```python
from build123d import *
from build123d.topology import SkipClean

# Parameters (mm, degrees)
SKETCH1_R      = 10.5
EXTRUDE1_DEPTH = 1
EXTRUDE6_DEPTH = 3
SKETCH9_R      = 5.75
EXTRUDE9_DEPTH = 0.25
SKETCH7_R      = 4.9
EXTRUDE7_DEPTH = 2.366666667
SKETCH8_R      = 2
EXTRUDE8_DEPTH = 17.156560415
FILLET2_R      = 0.4
CHAMFER2_SIZE  = 1
FILLET3_R      = 1.5


with BuildPart() as part:
    # Sketch1 → Extrude1 (new body)
    with BuildSketch(Plane(origin=(0, 0, 0), x_dir=(1, 0, 0), z_dir=(0, 1, 0))):
        with Locations(Location((0, 0, 0), (0, 0, 270))):
            Circle(SKETCH1_R)
    extrude(amount=EXTRUDE1_DEPTH)

    # Sketch6 → Extrude6 (add)
    with SkipClean():  # the faces are left unmerged after this step: merging them gives an invalid solid
        with BuildSketch(Plane(origin=(0, 1, 0), x_dir=(1, 0, 0), z_dir=(0, 1, 0))):
            with BuildLine():
                Line((-2, 10.307764064), (-2, 8.209902557))
                ThreePointArc((-2, 8.209902557), (-5.975052301, 5.975052301), (-8.209902557, 2))
                Line((-8.209902557, 2), (-10.307764064, 2))
                ThreePointArc((-10.307764064, 2), (-7.424621202, 7.424621202), (-2, 10.307764064))
            make_face()
            with BuildLine():
                Line((2, 10.307764064), (2, 8.209902557))
                ThreePointArc((2, 8.209902557), (5.975052301, 5.975052301), (8.209902557, 2))
                Line((8.209902557, 2), (10.307764064, 2))
                ThreePointArc((10.307764064, 2), (7.424621202, 7.424621202), (2, 10.307764064))
            make_face()
            with BuildLine():
                Line((10.307764064, -2), (8.209902557, -2))
                ThreePointArc((8.209902557, -2), (5.975052301, -5.975052301), (2, -8.209902557))
                Line((2, -8.209902557), (2, -10.307764064))
                ThreePointArc((2, -10.307764064), (7.424621202, -7.424621202), (10.307764064, -2))
            make_face()
            with BuildLine():
                Line((-2, -10.307764064), (-2, -8.209902557))
                ThreePointArc((-2, -8.209902557), (-5.975052301, -5.975052301), (-8.209902557, -2))
                Line((-8.209902557, -2), (-10.307764064, -2))
                ThreePointArc((-10.307764064, -2), (-7.424621202, -7.424621202), (-2, -10.307764064))
            make_face()
        extrude(amount=EXTRUDE6_DEPTH)

    # Sketch9 → Extrude9 (cut)
    with SkipClean():  # the faces are left unmerged after this step: merging them gives an invalid solid
        with BuildSketch(Plane(origin=(0, 1, 0), x_dir=(1, 0, 0), z_dir=(0, 1, 0))):
            with Locations(Location((0, 0, 0), (0, 0, 270))):
                Circle(SKETCH9_R)
        extrude(amount=-EXTRUDE9_DEPTH, mode=Mode.SUBTRACT)

    # Sketch7 → Extrude7 (add)
    with SkipClean():  # the faces are left unmerged after this step: merging them gives an invalid solid
        with BuildSketch(Plane.XZ):
            with Locations(Location((0, 0, 0), (0, 0, 270))):
                Circle(SKETCH7_R)
        extrude(amount=EXTRUDE7_DEPTH)

    # Sketch8 → Extrude8 (cut, through all)
    with SkipClean():  # the faces are left unmerged after this step: merging them gives an invalid solid
        with BuildSketch(Plane.XZ.offset(2.366666667)):
            with Locations(Location((0, 0, 0), (0, 0, 270))):
                Circle(SKETCH8_R)
        extrude(amount=-EXTRUDE8_DEPTH, mode=Mode.SUBTRACT)

    # Fillet2
    fillet2_edges = [part.edges().sort_by_distance(p)[0] for p in [
        (5.975052301, 4, -5.975052301),
        (5.975052301, 4, 5.975052301),
        (-5.975052301, 4, 5.975052301),
        (0, -2.366666667, 4.9),
        (-5.975052301, 4, -5.975052301),
    ]]
    fillet(fillet2_edges, radius=FILLET2_R)

    # Chamfer2
    chamfer2_edges = [part.edges().sort_by_distance(p)[0] for p in [
        (0, -2.366666667, 2),
    ]]
    chamfer(chamfer2_edges, length=CHAMFER2_SIZE)

    # Fillet3
    # the kernel refuses this fillet: 1.5 mm, written as the material it adds along each edge
    with BuildSketch(Plane(origin=(2, 1, -14.057764064), x_dir=(-1, 0, 0), z_dir=(0, 0, 1))) as fillet3_piece_1_section:
        with BuildLine():
            CenterArc((FILLET3_R, -FILLET3_R), FILLET3_R, 90, 90)
            Line((0, -FILLET3_R), (0, 0))
            Line((0, 0), (FILLET3_R, 0))
        make_face()
    fillet3_piece_1 = extrude(amount=9.597861507, mode=Mode.PRIVATE)
    fillet3_piece_1 = fillet3_piece_1 & Plane(origin=(0, 1.340711746, 0), x_dir=(0, 0, 1), z_dir=(0, -1, 0)) * Cylinder(10.5, 26, mode=Mode.PRIVATE)
    fillet3_piece_1 = fillet3_piece_1 - Plane(origin=(0, 1.340711746, 0), x_dir=(0.23668639053254556, 0, -0.9715861014530186), z_dir=(0, -1, 0)) * Cylinder(8.45, 26, mode=Mode.PRIVATE)
    with BuildSketch(Plane(origin=(4.459902557, 1, -2), x_dir=(0, 0, 1), z_dir=(1, 0, 0))) as fillet3_piece_2_section:
        with BuildLine():
            CenterArc((FILLET3_R, -FILLET3_R), FILLET3_R, 90, 90)
            Line((0, -FILLET3_R), (0, 0))
            Line((0, 0), (FILLET3_R, 0))
        make_face()
    fillet3_piece_2 = extrude(amount=9.597861507, mode=Mode.PRIVATE)
    fillet3_piece_2 = fillet3_piece_2 & Plane(origin=(0, 1.34071094, 0), x_dir=(0, 0, 1), z_dir=(0, -1, 0)) * Cylinder(10.5, 26, mode=Mode.PRIVATE)
    fillet3_piece_2 = fillet3_piece_2 - Plane(origin=(0, 1.34071094, 0), x_dir=(0.23668639053254556, 0, -0.9715861014530186), z_dir=(0, -1, 0)) * Cylinder(8.45, 26, mode=Mode.PRIVATE)
    with BuildSketch(Plane(origin=(14.057764064, 1, 2), x_dir=(0, 0, -1), z_dir=(-1, 0, 0))) as fillet3_piece_3_section:
        with BuildLine():
            CenterArc((FILLET3_R, -FILLET3_R), FILLET3_R, 90, 90)
            Line((0, -FILLET3_R), (0, 0))
            Line((0, 0), (FILLET3_R, 0))
        make_face()
    fillet3_piece_3 = extrude(amount=9.597861507, mode=Mode.PRIVATE)
    fillet3_piece_3 = fillet3_piece_3 & Plane(origin=(0, 1.340711718, 0), x_dir=(0, 0, 1), z_dir=(0, -1, 0)) * Cylinder(10.5, 26, mode=Mode.PRIVATE)
    fillet3_piece_3 = fillet3_piece_3 - Plane(origin=(0, 1.340711718, 0), x_dir=(0.9715861014530187, 0, 0.2366863905325454), z_dir=(0, -1, 0)) * Cylinder(8.45, 26, mode=Mode.PRIVATE)
    with BuildSketch(Plane(origin=(2, 1, 4.459902557), x_dir=(-1, 0, 0), z_dir=(0, 0, 1))) as fillet3_piece_4_section:
        with BuildLine():
            CenterArc((FILLET3_R, -FILLET3_R), FILLET3_R, 90, 90)
            Line((0, -FILLET3_R), (0, 0))
            Line((0, 0), (FILLET3_R, 0))
        make_face()
    fillet3_piece_4 = extrude(amount=9.597861507, mode=Mode.PRIVATE)
    fillet3_piece_4 = fillet3_piece_4 & Plane(origin=(0, 1.34071094, 0), x_dir=(0, 0, 1), z_dir=(0, -1, 0)) * Cylinder(10.5, 26, mode=Mode.PRIVATE)
    fillet3_piece_4 = fillet3_piece_4 - Plane(origin=(0, 1.34071094, 0), x_dir=(0.9715861014530187, 0, 0.2366863905325454), z_dir=(0, -1, 0)) * Cylinder(8.45, 26, mode=Mode.PRIVATE)
    with BuildSketch(Plane(origin=(-2, 1, 14.057764064), x_dir=(1, 0, 0), z_dir=(0, 0, -1))) as fillet3_piece_5_section:
        with BuildLine():
            CenterArc((FILLET3_R, -FILLET3_R), FILLET3_R, 90, 90)
            Line((0, -FILLET3_R), (0, 0))
            Line((0, 0), (FILLET3_R, 0))
        make_face()
    fillet3_piece_5 = extrude(amount=9.597861507, mode=Mode.PRIVATE)
    fillet3_piece_5 = fillet3_piece_5 & Plane(origin=(0, 1.340711184, 0), x_dir=(0, 0, 1), z_dir=(0, -1, 0)) * Cylinder(10.5, 26, mode=Mode.PRIVATE)
    fillet3_piece_5 = fillet3_piece_5 - Plane(origin=(0, 1.340711184, 0), x_dir=(-0.2366863905325458, 0, 0.9715861014530186), z_dir=(0, -1, 0)) * Cylinder(8.45, 26, mode=Mode.PRIVATE)
    with BuildSketch(Plane(origin=(-4.459902557, 1, 2), x_dir=(0, 0, -1), z_dir=(-1, 0, 0))) as fillet3_piece_6_section:
        with BuildLine():
            CenterArc((FILLET3_R, -FILLET3_R), FILLET3_R, 90, 90)
            Line((0, -FILLET3_R), (0, 0))
            Line((0, 0), (FILLET3_R, 0))
        make_face()
    fillet3_piece_6 = extrude(amount=9.597861507, mode=Mode.PRIVATE)
    fillet3_piece_6 = fillet3_piece_6 & Plane(origin=(0, 1.34071094, 0), x_dir=(0, 0, 1), z_dir=(0, -1, 0)) * Cylinder(10.5, 26, mode=Mode.PRIVATE)
    fillet3_piece_6 = fillet3_piece_6 - Plane(origin=(0, 1.34071094, 0), x_dir=(-0.2366863905325458, 0, 0.9715861014530186), z_dir=(0, -1, 0)) * Cylinder(8.45, 26, mode=Mode.PRIVATE)
    with BuildSketch(Plane(origin=(-4.459902557, 1, -2), x_dir=(0, 0, 1), z_dir=(-1, 0, 0))) as fillet3_piece_7_section:
        with BuildLine():
            CenterArc((FILLET3_R, FILLET3_R), FILLET3_R, 180, 90)
            Line((0, FILLET3_R), (0, 0))
            Line((0, 0), (FILLET3_R, 0))
        make_face()
    fillet3_piece_7 = extrude(amount=9.597861507, mode=Mode.PRIVATE)
    fillet3_piece_7 = fillet3_piece_7 & Plane(origin=(0, 1.340712249, 0), x_dir=(0, 0, 1), z_dir=(0, -1, 0)) * Cylinder(10.5, 26, mode=Mode.PRIVATE)
    fillet3_piece_7 = fillet3_piece_7 - Plane(origin=(0, 1.340712249, 0), x_dir=(-0.23668639053254495, 0, -0.9715861014530188), z_dir=(0, -1, 0)) * Cylinder(8.45, 26, mode=Mode.PRIVATE)
    with BuildSketch(Plane(origin=(-2, 1, -14.057764064), x_dir=(1, 0, 0), z_dir=(0, 0, 1))) as fillet3_piece_8_section:
        with BuildLine():
            CenterArc((FILLET3_R, FILLET3_R), FILLET3_R, 180, 90)
            Line((0, FILLET3_R), (0, 0))
            Line((0, 0), (FILLET3_R, 0))
        make_face()
    fillet3_piece_8 = extrude(amount=9.597861507, mode=Mode.PRIVATE)
    fillet3_piece_8 = fillet3_piece_8 & Plane(origin=(0, 1.340709875, 0), x_dir=(0, 0, 1), z_dir=(0, -1, 0)) * Cylinder(10.5, 26, mode=Mode.PRIVATE)
    fillet3_piece_8 = fillet3_piece_8 - Plane(origin=(0, 1.340709875, 0), x_dir=(-0.23668639053254495, 0, -0.9715861014530188), z_dir=(0, -1, 0)) * Cylinder(8.45, 26, mode=Mode.PRIVATE)
    add([fillet3_piece_1, fillet3_piece_2, fillet3_piece_3, fillet3_piece_4, fillet3_piece_5, fillet3_piece_6, fillet3_piece_7, fillet3_piece_8])


solid = part.part
```
Build history of the part. All positions in model axes, mm. A direction names the side the tool comes from. Coordinates: 2 decimals unless noted, no trailing zeros. Order: outer loops, then holes, each group sorted by start corner. A loop starts at its lowest first (then second) coordinate and runs counter-clockwise, first axis right, second up. Notation, with made-up numbers: (10.25, -4) -> (44.25, -4) arc R21 cw to (44.25, 11) -> close; hole circle Ø8 at (59.5, 82). An arc over 180 degrees is marked (long way). Answer in a Markdown table with one row per item. Add a question column.
Q1. Mould opens along Z. For faces 1 (the face through (9.36, 1.43, 1.55)), 2 (the face through (1.55, 1.43, 9.33)) say: +Z half, -Z half, draft (parallel to the pull), parting line (faces both ways), or undercut.
Q2. Band-saw the part on C-C, the plane y = -0.25. List the corners of the cut face in (x, z).
Q3. Which spindle directions (+Z, -Z, +X, -X, +Y, -Y) get a long thin tool onto all of the face, cutting with end or side? Do faces 3 (the face through (9.33, 1.43, -1.55)), 4 (the face through (-2, 0, 5)), 5 (the face through (0.1, 0.75, 2.5)). Say none if no direction does.
Q4. Band-saw the part on A-A, the plane z = 0. List the corners of the cut face in (x, y), then the cut area to 3 significant figures.
Q5. Wall check: line 1 along X through (y, z) = (0.9, 0); line 2 along X through (y, z) = (-0.3, 0); line 3 along Y through (x, z) = (7.25, -6.75). Give the ranges that are in metal, low to high. Write a range as [from, to].
Q6. Drop flat-ended pins along their axis: pin 1 (1.7 mm diameter, centred on y = 3.5, z = -9.5, fed in from +X); pin 2 (3.5 mm diameter, centred on x = 1, z = -0.5, fed in from +Y); pin 3 (1.2 mm diameter, centred on y = 3.5, z = -9, fed in from -X); pin 4 (3.5 mm diameter, centred on x = 0, z = 0, fed in from -Y). Give the stop position or say it passes through.
Q7. Band-saw the part on B-B, the plane x = 0. List the corners of the cut face in (y, z), then the cut area to 3 significant figures.
Answers follow:
| question | item | result |
|---|---|---|
| 1 | face 1 | undercut |
| 1 | face 2 | draft |
| 2 | outline | circle Ø9.8 at (0, 0); hole circle Ø4 at (0, 0) |
| 3 | face 3 | +X, -X, +Y |
| 3 | face 4 | -Y |
| 3 | face 5 | +Y |
| 4 | outline | (-10.5, 0) -> (-4.9, 0) -> (-4.9, -1.97) arc R0.4 ccw to (-4.5, -2.37) -> (-3, -2.37) -> (-2, -1.37) -> (-2, 0.75) -> (-5.75, 0.75) -> (-5.75, 1) -> (-10.5, 1) -> close; (2, -1.37) -> (3, -2.37) -> (4.5, -2.37) arc R0.4 ccw to (4.9, -1.97) -> (4.9, 0) -> (10.5, 0) -> (10.5, 1) -> (5.75, 1) -> (5.75, 0.75) -> (2, 0.75) -> close |
| 4 | area | 27.8 mm^2 |
| 5 | line 1 | [-10.5, -5.75], [5.75, 10.5] |
| 5 | line 2 | [-4.9, -2], [2, 4.9] |
| 5 | line 3 | [0, 4] |
| 6 | pin 1 | x = 5.95 |
| 6 | pin 2 | y = 0.75 |
| 6 | pin 3 | x = -6.3 |
| 6 | pin 4 | through |
| 7 | outline | (-2.37, -4.5) arc R0.4 ccw to (-1.97, -4.9) -> (0, -4.9) -> (0, -10.5) -> (1, -10.5) -> (1, -5.75) -> (0.75, -5.75) -> (0.75, -2) -> (-1.37, -2) -> (-2.37, -3) -> close; (-2.37, 3) -> (-1.37, 2) -> (0.75, 2) -> (0.75, 5.75) -> (1, 5.75) -> (1, 10.5) -> (0, 10.5) -> (0, 4.9) -> (-1.97, 4.9) arc R0.4 ccw to (-2.37, 4.5) -> close |
| 7 | area | 27.8 mm^2 |
